Autodesk Inventor part; units mm, degrees
ref_plane "YZ Plane" through (0, 0, 0) normal (1, 0, 0) x (0, 1, 0)
ref_plane "XZ Plane" through (0, 0, 0) normal (0, 1, 0) x (-1, 0, 0)
ref_plane "XY Plane" through (0, 0, 0) normal (0, 0, 1) x (1, 0, 0)
sketch "スケッチ1" plane through (0, 0, 0) normal (0, 1, 0) x (-1, 0, 0)
  line L0 (0, 0) -> (6, 0)
  line L1 (0, -44) -> (0, 0)
  line L2 (6, 0) -> (6, -8)
  line L3 (6, -44) -> (6, -36)
  line L4 (6, -36) -> (16, -36)
  line L5 (6, -8) -> (16, -8)
  line L6 (6, -44) -> (0, -44)
  line L7 (16, -8) -> (20, -15)
  line L8 (16, -36) -> (20, -29)
  line L9 (20, -15) -> (20, -29)
  point P0 (0, -22)
  point P1 (10, -14.5)
  point P2 (10, -29.5)
  dimension "d2" = 8
  dimension "d3" = 6
  dimension "d4" = 8
  dimension "d5" = 6
  dimension "d9" = 10
  dimension "d10" = 10
  dimension "d11" = 10
extrude "押し出し1" add sketch "スケッチ1" along normal blind 6
sketch "スケッチ2" plane through (0, 6, 0) normal (0, 1, 0) x (1, 0, 0)
  line L0 (0, 0) -> (0, 44)
  line L1 (-16, 8) -> (-6, 8)
  line L2 (-6, 36) -> (-16, 36)
  point P0 (-10, 14.5)
  point P1 (-10, 29.5)
  dimension "d17" = 10
  dimension "d18" = 6.5
  dimension "d19" = 10
  dimension "d20" = 6.5
hole "穴1" at (-10, 6, -14.5) at (-10, 6, -29.5) direction (0, -1, 0) diameter 3.2 end through all
fillet "フィレット1" radius 3 2 edges at (-16, 3, -8) (-16, 3, -36)
fillet "フィレット2" radius 3 2 edges at (-20, 3, -29) (-20, 3, -15)
sketch "スケッチ3" plane through (0, 6, 0) normal (0, 1, 0) x (1, 0, 0)
  arc A0 (-20, 15.7967) -> (-19.6047, 14.3083) centre (-17, 15.7967) ccw
  line L0 (-19.6047, 14.3083) -> (-10.1295, 8)
  line L1 (-14.259, 8) -> (-6, 8)
  line L2 (-20, 28.2033) -> (-20, 15.7967)
  line L3 (-20, 22) -> (-17.294, 22)
  line L4 (-19.6047, 29.6917) -> (-10.1295, 36)
  line L5 (-10.1295, 8) -> (-16.3751, 6.1485)
  line L6 (-19.6047, 14.3083) -> (-16.8638, 9.5116)
  line L7 (-16.3751, 6.1485) -> (-19.6047, 14.3083)
  line L8 (-16.8638, 34.4884) -> (-19.6047, 29.6917)
  line L9 (-19.6047, 29.6917) -> (-16.8449, 39.8374)
  line L10 (-16.8449, 39.8374) -> (-10.1295, 36)
  point P0 (0, 0)
extrude "押し出し2" cut sketch "スケッチ3" against normal blind 10
properties part number "射出_ベルト固定" material "PET プラスチック"
Design review of the part built by this model. Coordinates are the model's own, in mm. A direction names the side the tool comes from. Give positions to 0.01 mm unless a question says otherwise; leave off trailing zeros. Write each loop counter-clockwise with the first axis right and the second up, starting at its lowest first coordinate (ties: lowest second). Pieces come first, ordered by that corner, then holes. Notation, with made-up numbers: (31.25, 27) -> (60.25, 27) arc R25 cw to (60.25, 43) -> close; hole circle Ø4 at (-22.75, 11.5). An arc over 180 degrees is marked (long way). Answer in a Markdown table with one row per item.
(1) Consider section C-C (z = -3). State the section outline as (x, y) points.
Results:
| item | result |
|---|---|
| outline | (-6, 0) -> (0, 0) -> (0, 6) -> (-6, 6) -> close |
(2) Consider section D-D (x = -19). State the section outline as (y, z) points.
Results:
| item | result |
|---|---|
| outline | (0, -30.09) -> (6, -30.09) -> (6, -13.91) -> (0, -13.91) -> close |
(3) Mouldability with a two-part tool opening along Z and no side actions: class faces 4 (the flat face through (-6, 3, -40)), 5 (the cylindrical face through (-10.07, 2.96, -16.1)), 6 (the cylindrical face through (-19.897, 3.042, -28.984)) as +Z half, -Z half, draft (parallel to the pull), parting line (faces both ways), or undercut.
Results:
| item | result |
|---|---|
| face 4 | draft |
| face 5 | undercut |
| face 6 | -Z half |
(4) To check wall thickness, follow probe 1 along Z at (x, y) = (-10, 2.2); probe 2 along X at (y, z) = (3.5, -37); probe 3 along X at (y, z) = (4.7, -14.5). State the ranges of each line that lie inside material, in increasing order.
Results:
| item | result |
|---|---|
| probe 1 | -36 to -31.1, -27.9 to -16.1, -12.9 to -8 |
| probe 2 | -6 to 0 |
| probe 3 | -19.71 to -11.6, -8.4 to 0 |
(5) For faces 1 (the flat face through (-6, 3, -4)), 2 (the flat face through (-3, 3, -44)), 3 (the flat face through (-8, 3, -36)), list the 3-axis set-ups (+Z, -Z, +X, -X, +Y, -Y) from which the entire face can be reached by the end or side of a thin tool; tool diameter is ignored.
Results:
| item | result |
|---|---|
| face 1 | +Z, -X, +Y, -Y |
| face 2 | -Z, +X, -X, +Y, -Y |
| face 3 | -Z, -X, +Y, -Y |
(6) Consider section B-B (y = 3.4). Count the separate pieces of the cut face and the enclosed holes in it, then the cut area to 3 significant figures.
Results:
| item | result |
|---|---|
| separate pieces | 1 |
| enclosed holes | 2 |
| area | 575 mm2 |
(7) Consider section A-A (x = -9). State the section outline as (y, z) points.
Results:
| item | result |
|---|---|
| outline | (0, -36) -> (6, -36) -> (6, -30.75) -> (0, -30.75) -> close; (0, -28.25) -> (6, -28.25) -> (6, -15.75) -> (0, -15.75) -> close; (0, -13.25) -> (6, -13.25) -> (6, -8) -> (0, -8) -> close |
(8) Clearance check with flat-ended pins moving along their axes: pin 1 (1 mm diameter, centred on x = -7.5, y = 3.5, fed in from -Z); pin 2 (1.8 mm diameter, centred on y = 4, z = -41, fed in from -X); pin 3 (3 mm diameter, centred on x = -10, z = -29.5, fed in from -Y); pin 4 (1.2 mm diameter, centred on x = -8.5, y = 2, fed in from +Z). State where each tip first meets the part, or that it passes through.
Results:
| item | result |
|---|---|
| pin 1 | z = -36 |
| pin 2 | x = -6 |
| pin 3 | through |
| pin 4 | z = -8 |
